Here's how the part is built. I have some questions about the finished solid (model axes, mm). Round coordinates to 2 decimals unless told otherwise and drop trailing zeros. Order: outer loops, then holes, each group sorted by start corner. A loop starts at its lowest first (then second) coordinate and runs counter-clockwise, first axis right, second up. Notation, with made-up numbers: (-36.5, -25) - (12.5, -25) arc R18 cw to (12.5, -11) - close; hole circle Ø7 at (51.5, 42.25). An arc over 180 degrees is marked (long way). Answer as a JSON object with one key per item and string values.
```python
from build123d import *

# Parameters (mm, degrees)
SKETCH1_R           = 61
SKETCH1_R_2         = 2.7
SKETCH1_W           = 10
SKETCH1_H           = 30
BOSS_EXTRUDE1_DEPTH = 2
SKETCH2_W           = 11.5
SKETCH2_H           = 7.5
CUT_EXTRUDE1_DEPTH  = 87.290208019
SKETCH5_R           = 1.6
SKETCH5_W           = 7
SKETCH5_H           = 7
SKETCH5_W_2         = 10
CUT_EXTRUDE4_DEPTH  = 87.290208019
SKETCH6_W           = 10
SKETCH6_H           = 8
SKETCH6_R           = 1.6
SKETCH6_W_2         = 2.1
CUT_EXTRUDE5_DEPTH  = 87.290208019
BOSS_EXTRUDE2_START = -2
BOSS_EXTRUDE2_DEPTH = 2
FILLET1_R           = 10


with BuildPart() as part:
    # Sketch1 → Boss-Extrude1 (new body)
    with BuildSketch(Plane(origin=(0, 0, 0), x_dir=(1, 0, 0), z_dir=(0, 1, 0))):
        with Locations(Location((0, 0, 0), (0, 0, 270))):
            Circle(SKETCH1_R)
        with Locations(Location((-27.5, 20, 0), (0, 0, 270))):
            Circle(SKETCH1_R_2, mode=Mode.SUBTRACT)
        with Locations(Location((-27.5, -10, 0), (0, 0, 270))):
            Circle(SKETCH1_R_2, mode=Mode.SUBTRACT)
        with Locations(Location((27.5, -10, 0), (0, 0, 90))):
            Circle(SKETCH1_R_2, mode=Mode.SUBTRACT)
        with Locations(Location((27.5, 20, 0), (0, 0, 90))):
            Circle(SKETCH1_R_2, mode=Mode.SUBTRACT)
        with Locations((44, 0)):
            Rectangle(SKETCH1_W, SKETCH1_H, mode=Mode.SUBTRACT)
        with Locations((-44, 0)):
            Rectangle(SKETCH1_W, SKETCH1_H, mode=Mode.SUBTRACT)
    extrude(amount=BOSS_EXTRUDE1_DEPTH)

    # Sketch2 → Cut-Extrude1 (cut, through all)
    with BuildSketch(Plane(origin=(0, 2, 0), x_dir=(1, 0, 0), z_dir=(0, 1, 0))):
        with Locations((0, 32.75)):
            Rectangle(SKETCH2_W, SKETCH2_H)
    extrude(amount=-CUT_EXTRUDE1_DEPTH, mode=Mode.SUBTRACT)

    # Sketch5 → Cut-Extrude4 (cut, through all)
    with BuildSketch(Plane.XZ):
        with Locations(Location((42, -28.871979931, 0), (0, 0, 270))):
            Circle(SKETCH5_R)
        with Locations(Location((-42, -28.871979931, 0), (0, 0, 90))):
            Circle(SKETCH5_R)
        with Locations(Location((-41.4, 30, 0), (0, 0, 270))):
            Circle(SKETCH5_R)
        with BuildLine():
            Line((-35, -26.871979931), (-25, -26.871979931))
            ThreePointArc((-25, -26.871979931), (-23, -28.871979931), (-25, -30.871979931))
            Line((-25, -30.871979931), (-35, -30.871979931))
            ThreePointArc((-35, -30.871979931), (-37, -28.871979931), (-35, -26.871979931))
        make_face()
        with BuildLine():
            Line((35, -26.871979931), (25, -26.871979931))
            ThreePointArc((25, -26.871979931), (23, -28.871979931), (25, -30.871979931))
            Line((25, -30.871979931), (35, -30.871979931))
            ThreePointArc((35, -30.871979931), (37, -28.871979931), (35, -26.871979931))
        make_face()
        with BuildLine():
            Line((-6, 19.2), (6, 19.2))
            ThreePointArc((6, 19.2), (10.2, 15), (6, 10.8))
            Line((6, 10.8), (-6, 10.8))
            ThreePointArc((-6, 10.8), (-10.2, 15), (-6, 19.2))
        make_face()
        with Locations((-28.5, -38.5)):
            Rectangle(SKETCH5_W, SKETCH5_H)
        with BuildLine():
            Line((39.8, 30), (39.8, 36))
            ThreePointArc((39.8, 36), (41.4, 37.6), (43, 36))
            Line((43, 36), (43, 30))
            ThreePointArc((43, 30), (41.4, 28.4), (39.8, 30))
        make_face()
        with Locations((30, -38.5)):
            Rectangle(SKETCH5_W_2, SKETCH5_H)
    extrude(amount=-CUT_EXTRUDE4_DEPTH, mode=Mode.SUBTRACT)

    # Sketch6 → Cut-Extrude5 (cut, through all)
    with BuildSketch(Plane(origin=(0, 2, 0), x_dir=(1, 0, 0), z_dir=(0, 1, 0))):
        with Locations((-44, 0)):
            Rectangle(SKETCH6_W, SKETCH6_H)
        with Locations(Location((-56, 0, 0), (0, 0, 270))):
            Circle(SKETCH6_R)
        with Locations((44, 0)):
            Rectangle(SKETCH6_W, SKETCH6_H)
        with Locations(Location((56, 0, 0), (0, 0, 270))):
            Circle(SKETCH6_R)
        with Locations(Location((-44, -21.5, 0), (0, 0, 270))):
            Circle(SKETCH6_R)
        with Locations(Location((0, 15, 0), (0, 0, 270))):
            Circle(SKETCH6_R)
        with Locations(Location((25, 50, 0), (0, 0, 270))):
            Circle(SKETCH6_R)
        with Locations(Location((0, 49, 0), (0, 0, 270))):
            Circle(SKETCH6_R)
        with Locations(Location((-25, 50, 0), (0, 0, 270))):
            Circle(SKETCH6_R)
        with Locations(Location((0, 0, 0), (0, 0, 270))):
            Circle(SKETCH6_R)
        with Locations((-37.95, 0)):
            Rectangle(SKETCH6_W_2, SKETCH6_H)
        with Locations((-50.05, 0)):
            Rectangle(SKETCH6_W_2, SKETCH6_H)
        with Locations((50.05, 0)):
            Rectangle(SKETCH6_W_2, SKETCH6_H)
        with Locations((37.95, 0)):
            Rectangle(SKETCH6_W_2, SKETCH6_H)
        with Locations(Location((44, -21.5, 0), (0, 0, 270))):
            Circle(SKETCH6_R)
    extrude(amount=-CUT_EXTRUDE5_DEPTH, mode=Mode.SUBTRACT)

    # Sketch7 → Boss-Extrude2 (add)
    with BuildSketch(Plane(origin=(0, 2, 0), x_dir=(1, 0, 0), z_dir=(0, 1, 0)).offset(BOSS_EXTRUDE2_START)):
        with BuildLine():
            Line((-55.670050575, -24.93682957), (-40, -61))
            Line((-40, -61), (0, -61))
            ThreePointArc((0, -61), (-33.165142818, -51.196418838), (-55.670050575, -24.93682957))
        make_face()
        with BuildLine():
            ThreePointArc((55.670050575, -24.93682957), (33.165142818, -51.196418838), (0, -61))
            Line((0, -61), (40, -61))
            Line((40, -61), (55.670050575, -24.93682957))
        make_face()
    extrude(amount=BOSS_EXTRUDE2_DEPTH)

    # Fillet1
    fillet1_edges = [part.edges().sort_by_distance(p)[0] for p in [
        (-40, 1, 61),
        (40, 1, 61),
    ]]
    fillet(fillet1_edges, radius=FILLET1_R)


solid = part.part
```
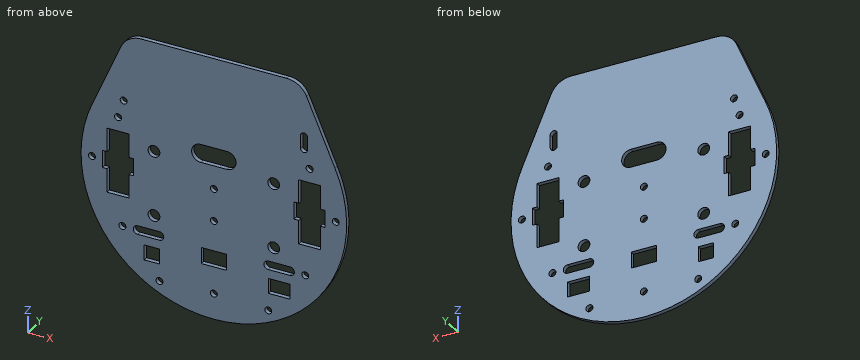
1. Imagine slicing it at C-C (y = 0.7). Give the number of separate pieces and of enclosed holes in the cut face, plus the area to 3 significant figures.
Responses:
{"separate pieces": "1", "enclosed holes": "25", "area": "10,900 mm2"}
2. Imagine slicing it at A-A (z = -33.5). List the corners of the cut face in (x, y) for me.
Responses:
{"outline": "(-50.98, 0) - (-5.75, 0) - (-5.75, 2) - (-50.98, 2) - close; (5.75, 0) - (50.98, 0) - (50.98, 2) - (5.75, 2) - close"}
3. Imagine slicing it at D-D (x = -53). List the corners of the cut face in (y, z) for me, plus the area to 3 significant figures.
Responses:
{"outline": "(0, -30.2) - (2, -30.2) - (2, 31.08) - (0, 31.08) - close", "area": "123 mm2"}
4. For P1, Ø1, axis at y = 1.5, z = -2.5, coming from the -X side; P2, Ø1, axis at x = -50, y = 1.5, coming from the -Z side; P3, Ø0.6, axis at x = -37.5, y = 0.5, coming from the +Z side, each with a flat end and sliding along its axis, tell me the tip position at first contact or that it passes through.
Responses:
{"P1": "x = -60.97", "P2": "z = -35.65", "P3": "z = 60.27"}
5. If I drill on L1, parallel to X at y = 1.4, z = -20; L2, parallel to X at y = 1.05, z = -49; L3, parallel to X at y = 1.1, z = -19, over which ranges is the centre line in solid material (lowest first)? Write a range as [from, to].
Responses:
{"L1": "[-57.63, -30.2], [-24.8, 24.8], [30.2, 57.63]", "L2": "[-36.33, -26.25], [-23.75, -1.6], [1.6, 23.75], [26.25, 36.33]", "L3": "[-57.97, -30.01], [-24.99, 24.99], [30.01, 57.97]"}
6. Imagine slicing it at B-B (x = 47). List the corners of the cut face in (y, z) for me.
Responses:
{"outline": "(0, -38.88) - (2, -38.88) - (2, -15) - (0, -15) - close; (0, 15) - (2, 15) - (2, 44.89) - (0, 44.89) - close"}
